Build history of the part. All positions in model axes, mm. Face numbers are marked on the shaded views. A direction names the side the tool comes from. Give positions to 0.01 mm unless a question says otherwise; leave off trailing zeros. Loops run counter-clockwise (first coordinate to the right, second up) from the corner with the lowest first, then second, coordinate; pieces in that order, holes last. Notation, with made-up numbers: M 24,84 L 81,84 A18 ccw 81,111 Z; hole C -5,84 d5. An arc over 180 degrees is marked long. Answer in a Markdown table with one row per item. Add a question column.
Autodesk Inventor part; units mm, degrees
ref_plane "Work Plane1" through (0, 15, 0) normal (0, 1, 0) x (-1, 0, 0)
ref_plane "YZ Plane" through (0, 0, 0) normal (1, 0, 0) x (0, 1, 0)
ref_plane "XY Plane" through (0, 0, 0) normal (0, 0, 1) x (1, 0, 0)
sketch "Sketch1" plane through (0, 0, 0) normal (0, 1, 0) x (-1, 0, 0)
  line L0 (24, 8) -> (27, 8)
  line L1 (27, 8) -> (27, 48)
  line L2 (27, 48) -> (25.5, 48)
  line L3 (25.5, 48) -> (25.5, 58)
  line L4 (26, 208) -> (25, 208)
  line L5 (25, 248) -> (25, 248)
  line L6 (0, 138) -> (0, -122.7414) construction
  line L7 (24, 8) -> (24, 0)
  line L8 (0, 98) -> (0, 0)
  line L9 (24, 0) -> (24.2, 0)
  line L10 (24.2, 0) -> (24.2, -4)
  line L11 (24.2, -4) -> (26, -4)
  line L12 (26, -4) -> (26, -54)
  line L13 (26, -54) -> (26.1, -54)
  line L14 (26.1, -54) -> (26.1, -134)
  line L15 (26.1, -134) -> (0, -134)
  line L16 (0, 0) -> (0, -134)
  line L17 (24, 0) -> (24.2, 0)
  line L18 (25.5, 58) -> (24.5, 58)
  line L19 (24.5, 58) -> (24.5, 98)
  line L20 (24.5, 98) -> (0, 98)
  dimension "d2" = 40
  dimension "d4" = 8
  dimension "d16" = 10
  dimension "d71" = 27
  dimension "d78" = 24
  dimension "d82" = 4
  dimension "d83" = 50
  dimension "d84" = 24.2
  dimension "d85" = 26.1
  dimension "d86" = 80
  dimension "d88" = 25.5
  dimension "d89" = 26
  dimension "d90" = 40
  dimension "d92" = 24.5
ref_plane "Work Plane1" through (0, 15, 0) normal (0, 1, 0) x (-1, 0, 0)
sketch "Sketch3" plane through (0, 15, 0) normal (0, 1, 0) x (-1, 0, 0)
  circle A0 centre (0, -79) radius 7
  point P0 (0, 0)
  dimension "d22" = 14
  dimension "d66" = 79
sketch "Sketch4" plane through (0, 0, 0) normal (1, 0, 0) x (0, 1, 0)
  circle A0 centre (0, -114) radius 7
  point P0 (0, 0)
  dimension "d28" = 14
  dimension "d67" = 114
revolve "Revolution1" add sketch "Sketch1" angle 360 about axis through (0, 0, 98) along (0, 0, -1)
extrude "Extrusion5" cut sketch "Sketch3" along normal blind 20 and the other way blind 45
extrude "Extrusion6" cut sketch "Sketch4" along normal blind 35 and the other way blind 30
chamfer "Chamfer3" distance 2 angle 45 1 edges at (27, 0, 8)
sketch "Sketch5" plane through (0, 0, 0) normal (0, 1, 0) x (-1, 0, 0)
  line L0 (24, 8) -> (24, 0)
  point P0 (0, 0)
sketch "Sketch6" plane through (0, 0, 0) normal (1, 0, 0) x (0, 1, 0)
  line L0 (0, 0) -> (-46.2751, 0) construction
equation "\"DiametroInterior\" = 52.2"
properties part number "Mangon_Conducido"
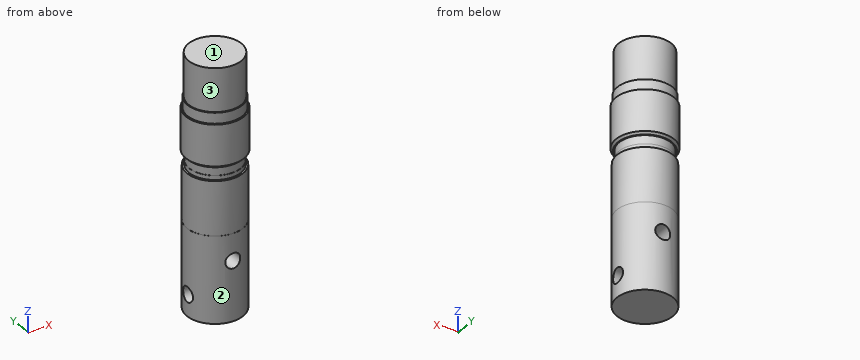
(1) Slice it at D-D, the plane z = -50.5. Give the cut face in (x, y), then the cut area to 3 significant figures.
(2) Wall check: line 1 (Z direction, x = 16, y = 0); line 2 (X direction, y = -13, z = -79); line 3 (Y direction, x = 7.5, z = -114). Give the ranges that are in metal, low to high.
(3) Slice it at C-C, the plane z = -114. Give the cut face in (x, y).
(4) Slice it at A-A, the plane y = 0. State how many separate pieces and enclosed holes the cut face has, then the cut area to 3 significant figures.
(5) Tool access for the marked faces 1, 2 and 3: list every direction of +Z, -Z, +X, -X, +Y, -Y with a clear straight run to the whole face (end or side of a thin tool).
(6) Pin check, flat tips, straight feed: pin 1 (2 mm diameter, centred on x = 10, z = -72, fed in from +Y); pin 2 (10 mm diameter, centred on y = -4, z = -94, fed in from -X); pin 3 (22.5 mm diameter, centred on x = 0, z = -79, fed in from +Y); pin 4 (12.5 mm diameter, centred on y = 0, z = -114, fed in from +X). Stop position of each tip, or through.
Solution:
| question | item | result |
|---|---|---|
| 1 | outline | C 0,0 d52 |
| 1 | area | 2,120 mm^2 |
| 2 | line 1 | -134 to -121, -107 to 98 |
| 2 | line 2 | -22.63 to -7, 7 to 22.63 |
| 2 | line 3 | -25 to -7, 7 to 25 |
| 3 | outline | M -25.14,-7 A26.1 ccw 25.14,-7 Z; M -25.14,7 L 25.14,7 A26.1 ccw Z |
| 4 | separate pieces | 2 |
| 4 | enclosed holes | 1 |
| 4 | area | 11,100 mm^2 |
| 5 | face 1 | +Z, +X, -X, +Y, -Y |
| 5 | face 2 | -Z |
| 5 | face 3 | +Z |
| 6 | pin 1 | y = 24.5 |
| 6 | pin 2 | x = -26.1 |
| 6 | pin 3 | y = 26.1 |
| 6 | pin 4 | through |
